```python
from build123d import *

# Parameters (mm, degrees)
SKETCH_1_W          = 5
SKETCH_1_H          = 5
EXTRUDE_1_DEPTH     = 58
SKETCH_1_5_W        = 6
SKETCH_1_5_H        = 6
EXTRUDE_2_DEPTH     = 3
SKETCH_1_3_R        = 1.35
CUT_EXTRUDE_1_DEPTH = 59.154965394
CUT_EXTRUDE_2_DEPTH = 2
SKETCH_3_R          = 0.3
CUT_EXTRUDE_3_DEPTH = 59.337380812
SKETCH_4_R          = 0.3
CUT_EXTRUDE_4_DEPTH = 59.337380911


with BuildPart() as part:
    # Sketch 1 → Extrude 1 (new body)
    with BuildSketch(Plane(origin=(0, 0, 0), x_dir=(1, 0, 0), z_dir=(0, 1, 0))):
        Rectangle(SKETCH_1_W, SKETCH_1_H)
    extrude(amount=EXTRUDE_1_DEPTH)

    # Sketch 1_5 → Extrude 2 (add)
    with BuildSketch(Plane(origin=(0, 0, 0), x_dir=(1, 0, 0), z_dir=(0, 1, 0))):
        Rectangle(SKETCH_1_5_W, SKETCH_1_5_H)
    extrude(amount=EXTRUDE_2_DEPTH)

    # Sketch 1_3 → Cut-Extrude 1 (cut, through all)
    with BuildSketch(Plane(origin=(0, 0, 0), x_dir=(1, 0, 0), z_dir=(0, 1, 0))):
        with Locations(Location((0, 0, 0), (0, 0, 90))):
            Circle(SKETCH_1_3_R)
    extrude(amount=CUT_EXTRUDE_1_DEPTH, mode=Mode.SUBTRACT)

    # Sketch 1_4 → Cut-Extrude 2 (cut)
    with BuildSketch(Plane(origin=(0, 0, 0), x_dir=(1, 0, 0), z_dir=(0, 1, 0))):
        Polygon((2.886751346, 0), (1.443375673, 2.5), (-1.443375673, 2.5), (-2.886751346, 0), (-1.443375673, -2.5), (1.443375673, -2.5), align=None)
    extrude(amount=CUT_EXTRUDE_2_DEPTH, mode=Mode.SUBTRACT)

    # Sketch 3 → Cut-Extrude 3 (cut, through all)
    with BuildSketch(Plane.XY.offset(2.5)):
        with Locations((0, 56)):
            Circle(SKETCH_3_R)
    extrude(amount=-CUT_EXTRUDE_3_DEPTH, mode=Mode.SUBTRACT)

    # Sketch 4 → Cut-Extrude 4 (cut, through all)
    with BuildSketch(Plane.ZY.offset(2.5)):
        with Locations((0, 56)):
            Circle(SKETCH_4_R)
    extrude(amount=-CUT_EXTRUDE_4_DEPTH, mode=Mode.SUBTRACT)


solid = part.part
```
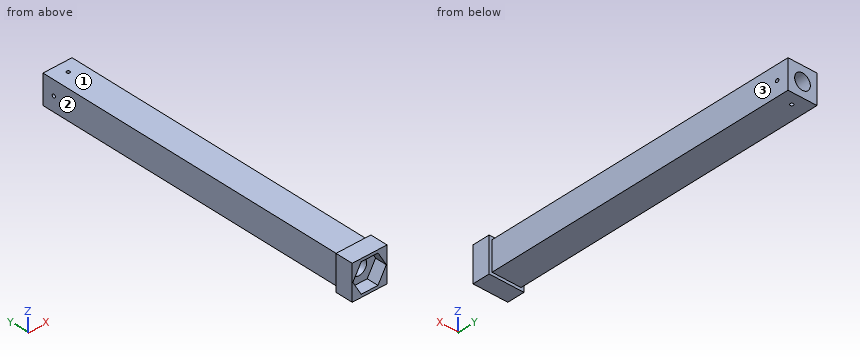
Can you work these out from the model? Positions are in its coordinate system, mm. Face numbers are marked on the shaded views. A direction names the side the tool comes from. Round coordinates to 2 decimals unless told otherwise and drop trailing zeros. Loops run counter-clockwise (first coordinate to the right, second up) from the corner with the lowest first, then second, coordinate; pieces in that order, holes last. Notation, with made-up numbers: M -9.75,66 L 8.25,66 A26 ccw 8.25,83 Z; hole C 88.25,78.25 d10. An arc over 180 degrees is marked long. Write item = value, one per line. Start each with the question number.
(1) Suppose I cut it at C-C on z = -2. Write out the boundary of the cut face in (x, y), plus the area to 3 significant figures.
(2) I need wall thicknesses on line 1 along X through (y, z) = (20, -0.1); line 2 along Y through (x, z) = (-1.6, 0); line 3 along Z through (x, y) = (-1.95, 56). Which ranges of each line are inside material? Lowest first, please.
(3) I'm going to push flat-ended pins straight in: P1, Ø1.8, axis at x = 1, z = 0, coming from the +Y side; P2, Ø1.5, axis at y = 31.5, z = 1, coming from the -X side; P3, Ø2, axis at y = 49, z = 0.5, coming from the +X side; P4, Ø2.5, axis at x = -0.5, y = 24, coming from the -Z side. Where does each tip first touch, or does it pass through?
(4) Suppose I cut it at B-B on y = 53. Write out the boundary of the cut face in (x, z).
(5) Suppose I cut it at A-A on z = 0.8. Write out the boundary of the cut face in (x, y), plus the area to 3 significant figures.
(6) Which directions (+Z, -Z, +X, -X, +Y, -Y) give clear straight access to the entire face, cutting with the end or side of a thin tool? Please do the marked faces 1, 2 and 3.
Answer block:
q1.outline = M -3,0 L -1.73,0 L -1.73,2 L 1.73,2 L 1.73,0 L 3,0 L 3,3 L 2.5,3 L 2.5,58 L -2.5,58 L -2.5,3 L -3,3 Z; hole C 0,56 d0.6
q1.area = 286 mm²
q2.line_1 = -2.5 to -1.35, 1.35 to 2.5
q2.line_2 = 2 to 55.7, 56.3 to 58
q2.line_3 = -2.5 to -0.3, 0.3 to 2.5
q3.P1 = 58
q3.P2 = -2.5
q3.P3 = 2.5
q3.P4 = -2.5
q4.outline = M -2.5,-2.5 L 2.5,-2.5 L 2.5,2.5 L -2.5,2.5 Z; hole C 0,0 d2.7
q5.outline = M -3,0 L -2.42,0 L -2.42,2 L -1.09,2 L -1.09,58 L -2.5,58 L -2.5,3 L -3,3 Z; M 1.09,2 L 2.42,2 L 2.42,0 L 3,0 L 3,3 L 2.5,3 L 2.5,58 L 1.09,58 Z
q5.area = 162 mm²
q6.face_1 = +Z, +X, -X, +Y
q6.face_2 = +Z, -Z, -X, +Y
q6.face_3 = +Z, -Z, +X, +Y
